Check sheet for the modelled part. Datum: model origin and axes. Units: mm. A direction names the side the tool comes from. Give positions to 0.01 mm unless a question says otherwise; leave off trailing zeros. Loops run counter-clockwise (first coordinate to the right, second up) from the corner with the lowest first, then second, coordinate; pieces in that order, holes last. Notation, with made-up numbers: (20.25, -3) - (27.25, -3) arc R19 ccw to (27.25, 32) - close; hole circle Ø9 at (26.25, 83.25). An arc over 180 degrees is marked (long way). Use one line per item in the form item = value.
from build123d import *

# Parameters (mm, degrees)
SKETCH1_R           = 1.5875
BOSS_EXTRUDE1_DEPTH = 2
SKETCH2_R           = 1.5875
BOSS_EXTRUDE2_DEPTH = 2.5
BOSS_EXTRUDE3_START = -3
SKETCH3_W           = 15.5
SKETCH3_H           = 3.5
BOSS_EXTRUDE3_DEPTH = 3
SKETCH4_R           = 1.5875
CUT_EXTRUDE1_DEPTH  = 5
CUT_EXTRUDE2_DEPTH  = 65.325422657


with BuildPart() as part:
    # Sketch1 → Boss-Extrude1 (new body)
    with BuildSketch(Plane(origin=(0, 0, 0), x_dir=(1, 0, 0), z_dir=(0, 1, 0))):
        with BuildLine():
            Line((-48, -42.4), (-43, -42.4))
            Line((-43, -42.4), (-36.009266938, -38.363898385))
            ThreePointArc((-36.009266938, -38.363898385), (-35.044543118, -37.964296695), (-34.009266938, -37.828))
            Line((-34.009266938, -37.828), (34.009266938, -37.828))
            ThreePointArc((34.009266938, -37.828), (35.044543118, -37.964296695), (36.009266938, -38.363898385))
            Line((36.009266938, -38.363898385), (43, -42.4))
            Line((43, -42.4), (48, -42.4))
            Line((48, -42.4), (48, 42.4))
            Line((48, 42.4), (43, 42.4))
            Line((43, 42.4), (36.009266938, 38.363898385))
            ThreePointArc((36.009266938, 38.363898385), (35.044543118, 37.964296695), (34.009266938, 37.828))
            Line((34.009266938, 37.828), (-34.009266938, 37.828))
            ThreePointArc((-34.009266938, 37.828), (-35.044543118, 37.964296695), (-36.009266938, 38.363898385))
            Line((-36.009266938, 38.363898385), (-43, 42.4))
            Line((-43, 42.4), (-48, 42.4))
            Line((-48, 42.4), (-48, -42.4))
        make_face()
        with Locations(Location((-12.7, -34.078, 0), (0, 0, 270))):
            Circle(SKETCH1_R, mode=Mode.SUBTRACT)
        with Locations(Location((12.7, -34.078, 0), (0, 0, 270))):
            Circle(SKETCH1_R, mode=Mode.SUBTRACT)
        with Locations(Location((-12.7, 34.078, 0), (0, 0, 270))):
            Circle(SKETCH1_R, mode=Mode.SUBTRACT)
        with Locations(Location((12.7, 34.078, 0), (0, 0, 270))):
            Circle(SKETCH1_R, mode=Mode.SUBTRACT)
        with Locations(Location((-42, 36.5, 0), (0, 0, 270))):
            Circle(SKETCH1_R, mode=Mode.SUBTRACT)
        with Locations(Location((42, 36.5, 0), (0, 0, 270))):
            Circle(SKETCH1_R, mode=Mode.SUBTRACT)
        with Locations(Location((42, -36.5, 0), (0, 0, 270))):
            Circle(SKETCH1_R, mode=Mode.SUBTRACT)
        with Locations(Location((-42, -36.5, 0), (0, 0, 270))):
            Circle(SKETCH1_R, mode=Mode.SUBTRACT)
        with BuildLine():
            Line((-38.65, 25.25), (-38.65, 9.75))
            ThreePointArc((-38.65, 9.75), (-41.825, 6.575), (-45, 9.75))
            Line((-45, 9.75), (-45, 25.25))
            ThreePointArc((-45, 25.25), (-41.825, 28.425), (-38.65, 25.25))
        make_face(mode=Mode.SUBTRACT)
        with BuildLine():
            Line((-38.65, -9.75), (-38.65, -25.25))
            ThreePointArc((-38.65, -25.25), (-41.825, -28.425), (-45, -25.25))
            Line((-45, -25.25), (-45, -9.75))
            ThreePointArc((-45, -9.75), (-41.825, -6.575), (-38.65, -9.75))
        make_face(mode=Mode.SUBTRACT)
        with BuildLine():
            Line((45, 25.25), (45, 9.75))
            ThreePointArc((45, 9.75), (41.825, 6.575), (38.65, 9.75))
            Line((38.65, 9.75), (38.65, 25.25))
            ThreePointArc((38.65, 25.25), (41.825, 28.425), (45, 25.25))
        make_face(mode=Mode.SUBTRACT)
        with BuildLine():
            Line((45, -9.75), (45, -25.25))
            ThreePointArc((45, -25.25), (41.825, -28.425), (38.65, -25.25))
            Line((38.65, -25.25), (38.65, -9.75))
            ThreePointArc((38.65, -9.75), (41.825, -6.575), (45, -9.75))
        make_face(mode=Mode.SUBTRACT)
    extrude(amount=BOSS_EXTRUDE1_DEPTH)

    # Sketch2 → Boss-Extrude2 (add)
    with BuildSketch(Plane(origin=(0, 2, 0), x_dir=(1, 0, 0), z_dir=(0, 1, 0))):
        with BuildLine():
            Line((48, -42.4), (48, 42.4))
            Line((48, 42.4), (43, 42.4))
            Line((43, 42.4), (36.009266938, 38.363898385))
            ThreePointArc((36.009266938, 38.363898385), (35.044543118, 37.964296695), (34.009266938, 37.828))
            Line((34.009266938, 37.828), (-34.009266938, 37.828))
            ThreePointArc((-34.009266938, 37.828), (-35.044543118, 37.964296695), (-36.009266938, 38.363898385))
            Line((-36.009266938, 38.363898385), (-43, 42.4))
            Line((-43, 42.4), (-48, 42.4))
            Line((-48, 42.4), (-48, -42.4))
            Line((-48, -42.4), (-43, -42.4))
            Line((-43, -42.4), (-36.009266938, -38.363898385))
            ThreePointArc((-36.009266938, -38.363898385), (-35.044543118, -37.964296695), (-34.009266938, -37.828))
            Line((-34.009266938, -37.828), (34.009266938, -37.828))
            ThreePointArc((34.009266938, -37.828), (35.044543118, -37.964296695), (36.009266938, -38.363898385))
            Line((36.009266938, -38.363898385), (43, -42.4))
            Line((43, -42.4), (48, -42.4))
        make_face()
        with Locations((-42, -36.5)):
            Circle(SKETCH2_R, mode=Mode.SUBTRACT)
        with Locations((-12.7, -34.078)):
            Circle(SKETCH2_R, mode=Mode.SUBTRACT)
        with Locations((12.7, -34.078)):
            Circle(SKETCH2_R, mode=Mode.SUBTRACT)
        with Locations((42, -36.5)):
            Circle(SKETCH2_R, mode=Mode.SUBTRACT)
        with Locations((-42, 36.5)):
            Circle(SKETCH2_R, mode=Mode.SUBTRACT)
        with Locations((-12.7, 34.078)):
            Circle(SKETCH2_R, mode=Mode.SUBTRACT)
        with BuildLine():
            Line((45, 9.75), (45, -9.75))
            Line((45, -9.75), (45, -25.25))
            ThreePointArc((45, -25.25), (44.07006403, -27.49506403), (41.825, -28.425))
            Line((41.825, -28.425), (-41.825, -28.425))
            ThreePointArc((-41.825, -28.425), (-44.07006403, -27.49506403), (-45, -25.25))
            Line((-45, -25.25), (-45, -9.75))
            Line((-45, -9.75), (-45, 9.75))
            Line((-45, 9.75), (-45, 25.25))
            ThreePointArc((-45, 25.25), (-44.07006403, 27.49506403), (-41.825, 28.425))
            Line((-41.825, 28.425), (41.825, 28.425))
            ThreePointArc((41.825, 28.425), (44.07006403, 27.49506403), (45, 25.25))
            Line((45, 25.25), (45, 9.75))
        make_face(mode=Mode.SUBTRACT)
        with Locations((12.7, 34.078)):
            Circle(SKETCH2_R, mode=Mode.SUBTRACT)
        with Locations((42, 36.5)):
            Circle(SKETCH2_R, mode=Mode.SUBTRACT)
    extrude(amount=BOSS_EXTRUDE2_DEPTH)

    # Sketch3 → Boss-Extrude3 (add)
    with BuildSketch(Plane(origin=(48, 0, 0), x_dir=(0, 0, -1), z_dir=(1, 0, 0)).offset(BOSS_EXTRUDE3_START)):
        with Locations((-17.5, 6.25)):
            Rectangle(SKETCH3_W, SKETCH3_H)
        with Locations((17.5, 6.25)):
            Rectangle(SKETCH3_W, SKETCH3_H)
    boss_extrude3 = extrude(amount=BOSS_EXTRUDE3_DEPTH)

    # Sketch4 → Cut-Extrude1 (cut)
    with BuildSketch(Plane(origin=(48, 0, 0), x_dir=(0, 0, -1), z_dir=(1, 0, 0))):
        with Locations((-17.5, 4)):
            Circle(SKETCH4_R)
        with Locations((17.5, 4)):
            Circle(SKETCH4_R)
    cut_extrude1 = extrude(amount=-CUT_EXTRUDE1_DEPTH, mode=Mode.SUBTRACT)

    # Mirror1: Boss-Extrude3, Cut-Extrude1 across plane
    add(boss_extrude3.mirror(Plane(origin=(0, 0, 0), x_dir=(0, 0, 1), z_dir=(1, 0, 0))))
    add(cut_extrude1.mirror(Plane(origin=(0, 0, 0), x_dir=(0, 0, 1), z_dir=(1, 0, 0))), mode=Mode.SUBTRACT)

    # Sketch5 → Cut-Extrude2 (cut, through all)
    with BuildSketch(Plane(origin=(0, 2, 0), x_dir=(1, 0, 0), z_dir=(0, 1, 0))):
        with BuildLine():
            Line((-26.127824556, -18.76552712), (-7.991792465, -2.216033952))
            ThreePointArc((-7.991792465, -2.216033952), (-7.013967909, 0), (-7.991792465, 2.216033952))
            Line((-7.991792465, 2.216033952), (-26.127824556, 18.76552712))
            ThreePointArc((-26.127824556, 18.76552712), (-29.361089111, 19.294172233), (-31.15, 16.549493168))
            Line((-31.15, 16.549493168), (-31.15, -16.549493168))
            ThreePointArc((-31.15, -16.549493168), (-29.361089111, -19.294172233), (-26.127824556, -18.76552712))
        make_face()
        with BuildLine():
            Line((19.87060859, 23.208966048), (2.022175444, 6.921912688))
            ThreePointArc((2.022175444, 6.921912688), (0, 6.137946639), (-2.022175444, 6.921912688))
            Line((-2.022175444, 6.921912688), (-19.87060859, 23.208966048))
            ThreePointArc((-19.87060859, 23.208966048), (-20.645583648, 26.509411856), (-17.848433147, 28.425))
            Line((-17.848433147, 28.425), (17.848433147, 28.425))
            ThreePointArc((17.848433147, 28.425), (20.645583648, 26.509411856), (19.87060859, 23.208966048))
        make_face()
        with BuildLine():
            Line((-19.87060859, -23.208966048), (-2.022175444, -6.921912688))
            ThreePointArc((-2.022175444, -6.921912688), (0, -6.137946639), (2.022175444, -6.921912688))
            Line((2.022175444, -6.921912688), (19.87060859, -23.208966048))
            ThreePointArc((19.87060859, -23.208966048), (20.645583648, -26.509411856), (17.848433147, -28.425))
            Line((17.848433147, -28.425), (-17.848433147, -28.425))
            ThreePointArc((-17.848433147, -28.425), (-20.645583648, -26.509411856), (-19.87060859, -23.208966048))
        make_face()
        with BuildLine():
            Line((7.991792465, 2.216033952), (26.127824556, 18.76552712))
            ThreePointArc((26.127824556, 18.76552712), (29.361089111, 19.294172233), (31.15, 16.549493168))
            Line((31.15, 16.549493168), (31.15, -16.549493168))
            ThreePointArc((31.15, -16.549493168), (29.361089111, -19.294172233), (26.127824556, -18.76552712))
            Line((26.127824556, -18.76552712), (7.991792465, -2.216033952))
            ThreePointArc((7.991792465, -2.216033952), (7.013967909, 0), (7.991792465, 2.216033952))
        make_face()
    extrude(amount=-CUT_EXTRUDE2_DEPTH, mode=Mode.SUBTRACT)


solid = part.part
Item 1: Thickness scan on L1, parallel to Z at x = 42, y = 1.5; L2, parallel to Z at x = 12.7, y = 3.3 (1 decimal); L3, parallel to Z at x = -42, y = 3.05. Record the ranges inside material, lowest first.
Answer block:
L1 = -41.82 to -38.09, -34.91 to -28.42, -6.58 to 6.58, 28.42 to 34.91, 38.09 to 41.82
L2 = -37.8 to -35.7, -32.5 to -28.4, 28.4 to 32.5, 35.7 to 37.8
L3 = -41.82 to -38.09, -34.91 to -28.42, 28.42 to 34.91, 38.09 to 41.82
Item 2: Section check B-B on x = 0. Record the boundary of the cut face in (y, z) (3 decimals).
Answer block:
outline = (0, -37.828) - (4.5, -37.828) - (4.5, -28.425) - (0, -28.425) - close; (0, -6.138) - (2, -6.138) - (2, 6.138) - (0, 6.138) - close; (0, 28.425) - (4.5, 28.425) - (4.5, 37.828) - (0, 37.828) - close
Item 3: Section check A-A on y = 6.75. Record the boundary of the cut face in (x, z), then the cut area to 3 significant figures.
Answer block:
outline = (-48, -25.25) - (-45, -25.25) - (-45, -9.75) - (-48, -9.75) - close; (-48, 9.75) - (-45, 9.75) - (-45, 25.25) - (-48, 25.25) - close; (45, -25.25) - (48, -25.25) - (48, -9.75) - (45, -9.75) - close; (45, 9.75) - (48, 9.75) - (48, 25.25) - (45, 25.25) - close
area = 186 mm2
Item 4: Gauge pin test, flat ends, axial feed: P1, Ø3, axis at x = -23, z = -29.5, coming from the +Y side; P2, Ø3.5, axis at x = 47, y = 6, coming from the -Z side; P3, Ø2.5, axis at x = -47, y = 6.5, coming from the -Z side; P4, Ø3.5, axis at x = 47, y = 6.5, coming from the +Z side. Record the tip position at first contact, or that the pin passes through.
Answer block:
P1 = 4.5
P2 = -42.4
P3 = -25.25
P4 = 25.25
Item 5: Access from +Z, -Z, +X, -X, +Y, -Y to the whole of each face (thin tool, end or side, straight path). Record for faces 1 (the face through (29.41, 1.01, 19.27)), 2 (the face through (46.521, 3.392, -18.966)), 3 (the face through (-46, 2, 42.4)), 4 (the face through (46, 4.5, 0)), 5 (the face through (45, 4, 0)).
Answer block:
face_1 = +Y, -Y
face_2 = +X, -X
face_3 = +Z, +X, -X, +Y, -Y
face_4 = +X, -X, +Y
face_5 = +Y
Item 6: Section check C-C on z = 14.5. Record the boundary of the cut face in (x, y).
Answer block:
outline = (-48, 0) - (-45, 0) - (-45, 8) - (-48, 8) - close; (-38.65, 0) - (-31.15, 0) - (-31.15, 2) - (-38.65, 2) - close; (-21.45, 0) - (-10.33, 0) - (-10.33, 2) - (-21.45, 2) - close; (10.33, 0) - (21.45, 0) - (21.45, 2) - (10.33, 2) - close; (31.15, 0) - (38.65, 0) - (38.65, 2) - (31.15, 2) - close; (45, 0) - (48, 0) - (48, 8) - (45, 8) - close
Item 7: Section check D-D on x = -15.5. Record the boundary of the cut face in (y, z) (3 decimals).
Answer block:
outline = (0, -37.828) - (4.5, -37.828) - (4.5, -28.425) - (0, -28.425) - close; (0, -19.221) - (2, -19.221) - (2, -9.067) - (0, -9.067) - close; (0, 9.067) - (2, 9.067) - (2, 19.221) - (0, 19.221) - close; (0, 28.425) - (4.5, 28.425) - (4.5, 37.828) - (0, 37.828) - close
Item 8: Mould release check, pull along X, two halves, no side actions. Record for faces 6 (the face through (-46, 8, -17)), 7 (the face through (48, 3, 1)), 8 (the face through (-35.03, 2.22, -37.96)): released by +X, released by -X, zero draft, split by the parting line, or undercut.
Answer block:
face_6 = zero draft
face_7 = released by +X
face_8 = undercut
